The listing builds one solid part. Answer for the finished solid, in the listing's coordinates (mm). Give positions to 0.01 mm unless a question says otherwise; leave off trailing zeros. Order: outer loops, then holes, each group sorted by start corner. A loop starts at its lowest first (then second) coordinate and runs counter-clockwise, first axis right, second up. Notation, with made-up numbers: (-36.75, 23) -> (14.25, 23) arc R27 cw to (14.25, 44) -> close; hole circle Ø11 at (66.5, -38.5). An arc over 180 degrees is marked (long way). Write item = value, one per line. Start each with the question number.
Autodesk Inventor part; units mm, degrees
ref_plane "YZ Plane" through (0, 0, 0) normal (1, 0, 0) x (0, 1, 0)
ref_plane "XZ Plane" through (0, 0, 0) normal (0, 1, 0) x (-1, 0, 0)
ref_plane "XY Plane" through (0, 0, 0) normal (0, 0, 1) x (1, 0, 0)
sketch "Sketch1" plane through (0, 0, 0) normal (0, 0, 1) x (1, 0, 0)
  line L0 (32.5, -15) -> (-32.5, -15)
  line L1 (-32.5, -15) -> (-32.5, 15)
  line L2 (-32.5, 15) -> (32.5, 15)
  line L3 (32.5, 15) -> (32.5, -15)
  line L4 (32.5, -15) -> (-32.5, 15) construction
  line L5 (-32.5, -15) -> (32.5, 15) construction
  circle A0 centre (0, 0) radius 1.25
  circle A1 centre (-30, 11) radius 1.3364
  circle A2 centre (25, 11.5385) radius 1.3533
  circle A3 centre (31.3333, -14.4615) radius 1.3333
  circle A4 centre (-30, -15) radius 1.3333
  dimension "d0" = 30
  dimension "d1" = 65
  dimension "d2" = 2.5
  dimension "d3" = 26
  dimension "d4" = 26
  dimension "d5" = 55
  dimension "d6" = 25
  dimension "d7" = 15
extrude "Plate1" add sketch "Sketch1" along normal blind 4 contours L0 A3 L3 | L0 A4 L1 L2 L3 A3 | L0 A4 picked at (30.9112, -14.2924) picked at (-29.6065, -14.7935)
sketch "Sketch2" plane through (0, 0, 4) normal (0, 0, 1) x (1, 0, 0)
  circle A0 centre (-29.8197, -12.1072) radius 1.6051
  circle A1 centre (28.6987, -12.1072) radius 1.4574
  point P0 (0, 0)
extrude "Extrusion1" cut sketch "Sketch2" against normal blind 5
sketch "Sketch3" plane through (0, 0, 4) normal (0, 0, 1) x (1, 0, 0)
  circle A0 centre (-27.5776, 6.8384) radius 0.7927
  circle A1 centre (-28.3703, -3.8115) radius 0.8238
  circle A2 centre (-16.143, -1.9058) radius 1.2074
  circle A3 centre (-11.7709, 11.3225) radius 1.1266
  circle A4 centre (6.0536, -6.6141) radius 1.4269
  circle A5 centre (14.7977, 6.8384) radius 1.466
  circle A6 centre (20.6272, -8.041) radius 1.4486
  point P0 (0, 0)
extrude "Extrusion2" cut sketch "Sketch3" against normal blind 5 contours A2 | A3 | A4 | A5 | A6
equation "\"d8\" = Thickness"
equation "\"BendRadius\" = Thickness"
equation "\"BendReliefWidth\" = Thickness"
equation "\"BendReliefDepth\" = 0.5 * Thickness"
equation "\"CornerReliefSize\" = 4 * Thickness"
equation "\"MinimumRemnant\" = 2 * Thickness"
equation "\"TransitionRadius\" = BendRadius"
equation "\"JacobiRadiusSize\" = BendRadius"
equation "\"GapSize\" = Thickness"
properties part number "rectanglar"
Item 1: A cutting plane is placed at C-C, the plane x = -30. Write down the section's boundary in (y, z).
Item 2: Consider L1, parallel to Y at x = 0, z = 2.6; L2, parallel to X at y = 11.25, z = 3.45; L3, parallel to Y at x = -16, z = 1.25. Determine where each line is inside the solid, lowest interval first. Write a range as from..to.
Item 3: The mould has two halves that part along X. Classify faces 1 (the flat face through (-32.5, 0, 2)), 2 (the flat face through (32.5, 0, 2)), 3 (the flat face through (0, 4, 4)), 4 (the cylindrical face through (7.37, -7.16, 2.03)): +X half, -X half, draft (parallel to the pull), parting line (faces both ways), or undercut.
Item 4: A cutting plane is placed at D-D, the plane z = 2.5. Count the separate pieces of the cut face and the enclosed holes in it, plus the area to 3 significant figures.
Item 5: A cutting plane is placed at A-A, the plane x = 25. Write down the section's boundary in (y, z), plus the area to 3 significant figures.
Item 6: Flat-ended cylindrical pins translate along their axes: pin 1 (3.5 mm diameter, centred on x = -30, y = 11, fed in from -Z); pin 2 (2.5 mm diameter, centred on x = -29.82, y = -12.11, fed in from -Z). Find the tip coordinate at first contact, or state that the pin passes through.
Item 7: A cutting plane is placed at B-B, the plane y = 0. Write down the section's boundary in (x, z).
Check values:
q1.outline = (-15, 0) -> (-13.7, 0) -> (-13.7, 4) -> (-15, 4) -> close; (-10.51, 0) -> (9.66, 0) -> (9.66, 4) -> (-10.51, 4) -> close; (12.34, 0) -> (15, 0) -> (15, 4) -> (12.34, 4) -> close
q2.L1 = -15..-1.25, 1.25..15
q2.L2 = -32.5..-31.31, -28.69..-12.9, -10.65..23.68, 26.32..32.5
q2.L3 = -15..-3.1, -0.71..15
q3.face_1 = -X half
q3.face_2 = +X half
q3.face_3 = draft
q3.face_4 = undercut
q4.separate_pieces = 1
q4.enclosed_holes = 10
q4.area = 1,890 mm^2
q5.outline = (-15, 0) -> (10.19, 0) -> (10.19, 4) -> (-15, 4) -> close; (12.89, 0) -> (15, 0) -> (15, 4) -> (12.89, 4) -> close
q5.area = 109 mm^2
q6.pin_1 = 0
q6.pin_2 = through
q7.outline = (-32.5, 0) -> (-1.25, 0) -> (-1.25, 4) -> (-32.5, 4) -> close; (1.25, 0) -> (32.5, 0) -> (32.5, 4) -> (1.25, 4) -> close
